```python
from build123d import *

# Parameters (mm, degrees)
SKETCH1_W                 = 220
SKETCH1_H                 = 220
SKETCH1_W_2               = 180
SKETCH1_H_2               = 180
EXTRUDE_THIN1_DEPTH       = 2
SKETCH2_R                 = 2
CUT_EXTRUDE1_DEPTH        = 10
LPATTERN1_COUNT           = 2
LPATTERN1_PITCH           = 98
LPATTERN1_COL_COUNT       = 2
LPATTERN1_COL_PITCH       = 98
LPATTERN2_COPY_1_SKETCH_R = 2
LPATTERN2_COPY_1_DEPTH    = 10
LPATTERN2_COPY_2_SKETCH_R = 2
LPATTERN2_COPY_2_DEPTH    = 10
LPATTERN2_COPY_3_SKETCH_R = 2
LPATTERN2_COPY_3_DEPTH    = 10
LPATTERN2_COPY_4_SKETCH_R = 2
LPATTERN2_COPY_4_DEPTH    = 10
LPATTERN3_COUNT           = 3
LPATTERN3_PITCH           = 196


with BuildPart() as part:
    # Sketch1 → Extrude-Thin1 (new body)
    with BuildSketch(Plane.XY):
        Rectangle(SKETCH1_W, SKETCH1_H)
        Rectangle(SKETCH1_W_2, SKETCH1_H_2, mode=Mode.SUBTRACT)
    extrude(amount=EXTRUDE_THIN1_DEPTH)

    # Sketch2 → Cut-Extrude1 (cut)
    with BuildSketch(Plane.XY.offset(2)):
        with Locations((0, 98)):
            Circle(SKETCH2_R)
    cut_extrude1 = extrude(amount=-CUT_EXTRUDE1_DEPTH, mode=Mode.SUBTRACT)

    # LPattern1: Cut-Extrude1 ×2
    with Locations(*[(i * LPATTERN1_PITCH, 0, 0) for i in range(1, LPATTERN1_COUNT)]):
        add(cut_extrude1, mode=Mode.SUBTRACT)

    # LPattern1 col: Cut-Extrude1 ×2
    with Locations(*[(-i * LPATTERN1_COL_PITCH, 0, 0) for i in range(1, LPATTERN1_COL_COUNT)]):
        add(cut_extrude1, mode=Mode.SUBTRACT)

    # LPattern2 copy 1 sketch → LPattern2 copy 1 (cut)
    with BuildSketch(Plane(origin=(98, -98, 2), x_dir=(1, 0, 0), z_dir=(0, 0, 1))):
        with Locations((0, 98)):
            Circle(LPATTERN2_COPY_1_SKETCH_R)
    extrude(amount=-LPATTERN2_COPY_1_DEPTH, mode=Mode.SUBTRACT)

    # LPattern2 copy 2 sketch → LPattern2 copy 2 (cut)
    with BuildSketch(Plane(origin=(98, -196, 2), x_dir=(1, 0, 0), z_dir=(0, 0, 1))):
        with Locations((0, 98)):
            Circle(LPATTERN2_COPY_2_SKETCH_R)
    extrude(amount=-LPATTERN2_COPY_2_DEPTH, mode=Mode.SUBTRACT)

    # LPattern2 copy 3 sketch → LPattern2 copy 3 (cut)
    with BuildSketch(Plane(origin=(-98, -98, 2), x_dir=(1, 0, 0), z_dir=(0, 0, 1))):
        with Locations((0, 98)):
            Circle(LPATTERN2_COPY_3_SKETCH_R)
    extrude(amount=-LPATTERN2_COPY_3_DEPTH, mode=Mode.SUBTRACT)

    # LPattern2 copy 4 sketch → LPattern2 copy 4 (cut)
    with BuildSketch(Plane(origin=(-98, -196, 2), x_dir=(1, 0, 0), z_dir=(0, 0, 1))):
        with Locations((0, 98)):
            Circle(LPATTERN2_COPY_4_SKETCH_R)
    extrude(amount=-LPATTERN2_COPY_4_DEPTH, mode=Mode.SUBTRACT)

    # LPattern3: Cut-Extrude1 ×3
    with Locations(*[(0, -i * LPATTERN3_PITCH, 0) for i in range(1, LPATTERN3_COUNT)]):
        add(cut_extrude1, mode=Mode.SUBTRACT)


solid = part.part
```
Build history of the part. All positions in model axes, mm. Give positions to 0.01 mm unless a question says otherwise; leave off trailing zeros. Order: outer loops, then holes, each group sorted by start corner. A loop starts at its lowest first (then second) coordinate and runs counter-clockwise, first axis right, second up. Notation, with made-up numbers: M 55,19 L 111,19 A27 ccw 111,48 Z; hole C -32,89.25 d1. An arc over 180 degrees is marked long. Write item = value, one per line. Start each with the question number.
(1) Slice it at C-C on z = 0.45. State how many separate pieces and enclosed holes the cut face has, plus the area to 3 significant figures.
(2) Pin check, flat tip, straight feed: pin 1 Ø3 at (x, y) = (98, 98) entering from -Z. Stop position of the tip, or through.
(3) Probe L1, parallel to Y at x = 98, z = 1.4; L2, parallel to Y at x = 0, z = 0.65; L3, parallel to X at y = 57, z = 0.6. List the from-to ranges inside material, lowest first. Write a range as [from, to].
(4) Slice it at A-A on x = -39. Write the cut outline in (y, z), plus the area to 3 significant figures.
Responses:
q1.separate_pieces = 1
q1.enclosed_holes = 9
q1.area = 15,900 mm2
q2.pin_1 = through
q3.L1 = [-110, -100], [-96, -2], [2, 96], [100, 110]
q3.L2 = [-110, -100], [-96, -90], [90, 96], [100, 110]
q3.L3 = [-110, -90], [90, 110]
q4.outline = M -110,0 L -90,0 L -90,2 L -110,2 Z; M 90,0 L 110,0 L 110,2 L 90,2 Z
q4.area = 80.0 mm2
